Can you work these out from the model? Positions are in its coordinate system, mm. Face numbers are marked on the shaded views. A direction names the side the tool comes from. Give positions to 0.01 mm unless a question says otherwise; leave off trailing zeros. Loops run counter-clockwise (first coordinate to the right, second up) from the corner with the lowest first, then second, coordinate; pieces in that order, holes last. Notation, with made-up numbers: (10, 0.25) -> (52, 0.25) arc R16 ccw to (52, 19.25) -> close; hole circle Ø7 at (57, 81.5). An arc over 180 degrees is marked (long way). Return JSON: item names as keys, results as strings. Group by question number.
Q1. Suppose I cut it at C-C, the plane y = 17. Please give me the cut outline in (x, z), and give its area (3 significant figures).
Q2. Suppose I cut it at B-B, the plane y = 35. Please give me the cut outline in (x, z).
Q3. Suppose I cut it at D-D, the plane x = 9.5. Please give me the cut outline in (y, z).
Q4. Which directions (+Z, -Z, +X, -X, +Y, -Y) give clear straight access to the entire face, cutting with the end or side of a thin tool? Please do the marked faces 1, 2 and 3.
Q5. Will these pins go through, and if not, where does the flat tip stop? pin 1 (3 mm diameter, centred on x = -20, y = 34.5, fed in from -Z); pin 2 (5 mm diameter, centred on x = 16.5, z = -4.5, fed in from +Y); pin 3 (4.5 mm diameter, centred on x = -21.5, y = 35, fed in from +Z); pin 4 (4 mm diameter, centred on y = 35, z = 5, fed in from -X).
Q6. I need wall thicknesses on line 1 along X through (y, z) = (9, 9); line 2 along Z through (x, y) = (19.75, 35); line 3 along Y through (x, z) = (-20, 22.5). Which ranges of each line are inside material? Lowest first, please. Write a range as [from, to].
Q7. Suppose I cut it at A-A, the plane x = 20. Please give me the cut outline in (y, z), and give its area (3 significant figures).
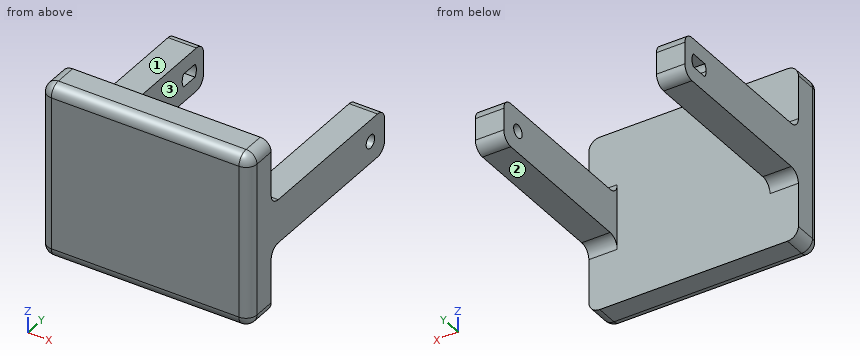
```python
from build123d import *

# Parameters (mm, degrees)
F0_W     = 6.5
F0_H     = 40
F1_DEPTH = 10
F4_DEPTH = 6.5
F2_R     = 1.5
F5_DEPTH = 6.5
F7_DEPTH = 15
F8_DEPTH = 15
F9_R     = 2.5


# Not quite as in the source:
# - a feature names something its author has since deleted; it is built from what else it names


with BuildPart() as f1:
    # F0 (on Top) → F1 (new body)
    with BuildSketch(Plane.XY):
        with Locations((-20.75, 20)):
            Rectangle(F0_W, F0_H)
        with Locations((20.75, 20)):
            Rectangle(F0_W, F0_H)
        Polygon((-17.5, 0), (-24, 0), (-24, -7.5), (24, -7.5), (24, 0), (17.5, 0), align=None)
    extrude(amount=F1_DEPTH)

    # F3 (on face) → F4 (cut, through all)
    with BuildSketch(Plane(origin=(-24, 0, 0), x_dir=(0, -1, 0), z_dir=(-1, 0, 0))):
        with BuildLine():
            ThreePointArc((-33, 3.5), (-32.6282917549, 4.209430585), (-32.5, 5))
            ThreePointArc((-32.5, 5), (-32.6282917549, 5.790569415), (-33, 6.5))
            Line((-33, 6.5), (-37, 6.5))
            ThreePointArc((-37, 6.5), (-37.5, 5), (-37, 3.5))
            Line((-37, 3.5), (-33, 3.5))
        make_face()
    extrude(amount=-F4_DEPTH, mode=Mode.SUBTRACT)

    # F2 (on face) → F5 (cut, through all)
    with BuildSketch(Plane.YZ.offset(24)):
        with Locations((35, 5)):
            Circle(F2_R)
    extrude(amount=-F5_DEPTH, mode=Mode.SUBTRACT)

    # F6 (on face) → F7 (join)
    with BuildSketch(Plane.XY.offset(10)):
        Polygon((-17.5, 0), (-24, 0), (-24, -7.5), (24, -7.5), (24, 0), (17.5, 0), align=None)
    extrude(amount=F7_DEPTH)

    # F0 (on Top) → F8 (join)
    with BuildSketch(Plane.XY):
        Polygon((-17.5, 0), (-24, 0), (-24, -7.5), (24, -7.5), (24, 0), (17.5, 0), align=None)
    extrude(amount=-F8_DEPTH)

    # F9
    f9_edges = [f1.edges().sort_by_distance(p)[0] for p in [
        (-24, -7.5, 5),
        (24, -7.5, 5),
        (-20.75, 40, 10),
        (-20.75, 40, 0),
        (20.75, 40, 10),
        (20.75, 40, 0),
        (0, -7.5, 25),
        (24, -3.75, 25),
        (-24, -3.75, 25),
        (-24, -3.75, -15),
        (24, -3.75, -15),
        (0, -7.5, -15),
        (20.75, 0, 10),
        (20.75, 0, 0),
        (-20.75, 0, 10),
        (-20.75, 0, 0),
    ]]
    fillet(f9_edges, radius=F9_R)


solid = f1.part
```
Ans:
{
 "1": {"outline": "(-24, 0) -> (-17.5, 0) -> (-17.5, 10) -> (-24, 10) -> close; (17.5, 0) -> (24, 0) -> (24, 10) -> (17.5, 10) -> close", "area": "130 mm^2"},
 "2": {"outline": "(-24, 0) -> (-17.5, 0) -> (-17.5, 3.5) -> (-24, 3.5) -> close; (-24, 6.5) -> (-17.5, 6.5) -> (-17.5, 10) -> (-24, 10) -> close; (17.5, 0) -> (24, 0) -> (24, 3.5) -> (17.5, 3.5) -> close; (17.5, 6.5) -> (24, 6.5) -> (24, 10) -> (17.5, 10) -> close"},
 "3": {"outline": "(-7.5, -12.5) arc R2.5 ccw to (-5, -15) -> (0, -15) -> (0, 25) -> (-5, 25) arc R2.5 ccw to (-7.5, 22.5) -> close"},
 "4": {"face 1": "+Z, +X, -X, +Y", "face 2": "-Z, +X, -X, +Y", "face 3": "+Z, -Z, +Y"},
 "5": {"pin 1": "stops at z = 0", "pin 2": "stops at y = 0.02", "pin 3": "stops at z = 10", "pin 4": "stops at x = -24"},
 "6": {"line 1": "x = [-24, -17.5], [17.5, 24]", "line 2": "z = [0, 3.5], [6.5, 10]", "line 3": "y = [-7.5, 0]"},
 "7": {"outline": "(-7.5, -12.5) arc R2.5 ccw to (-5, -15) -> (0, -15) -> (0, -2.5) arc R2.5 cw to (2.5, 0) -> (37.5, 0) arc R2.5 ccw to (40, 2.5) -> (40, 7.5) arc R2.5 ccw to (37.5, 10) -> (2.5, 10) arc R2.5 cw to (0, 12.5) -> (0, 25) -> (-5, 25) arc R2.5 ccw to (-7.5, 22.5) -> close; hole circle Ø3 at (35, 5)", "area": "690 mm^2"}
}
